Answer from the drawing. Dimensions are ordinates in mm from the lowest x, y and z of the part. A direction names the side the tool comes from. Coordinates: 2 decimals unless noted, no trailing zeros. Write each loop counter-clockwise with the first axis right and the second up, starting at its lowest first coordinate (ties: lowest second). Pieces come first, ordered by that corner, then holes. Notation, with made-up numbers: (40, 11.25) - (73, 11.25) arc R7 ccw to (73, 16.25) - close; hole circle Ø1 at (66, -31). An arc over 180 degrees is marked (long way). Use one line per item in the form item = value. Start each with the question number.
Item 1: Consider probe 1 along X at (y, z) = (28.35, 15); probe 2 along X at (y, z) = (17.5, 4.5); probe 3 along Y at (x, z) = (10.25, 26). Determine where each line is inside the solid, lowest interval first.
Item 2: Determine the mould class of the marked faces 1, 2 and 3 for opening direction X: released by +X, released by -X, zero draft, split by the parting line, or undercut.
Item 3: A cutting plane is placed at A-A (y = 17). Write down the section's boundary in (x, z), then the cut area to 3 significant figures.
Item 4: A cutting plane is placed at C-C (z = 15). Write down the section's boundary in (x, y), then the cut area to 4 significant figures.
Item 5: For the marked faces 4 and 5, determine the directions among +Z, -Z, +X, -X, +Y, -Y from which every point of the face is accessible in a straight line to the end or side of a thin tool.
Item 6: Given pin 1 (8 mm diameter, centred on y = 8, z = 15.5, fed in from +X); pin 2 (8 mm diameter, centred on x = 11, z = 12.5, fed in from -Y), each flat-ended and moving along its own axis, determine where each tip first touches the part or whether it passes through.
Item 7: A cutting plane is placed at D-D (z = 22). Write down the section's boundary in (x, y), then the cut area to 3 significant figures.
Item 8: A cutting plane is placed at B-B (x = 15). Write down the section's boundary in (y, z).
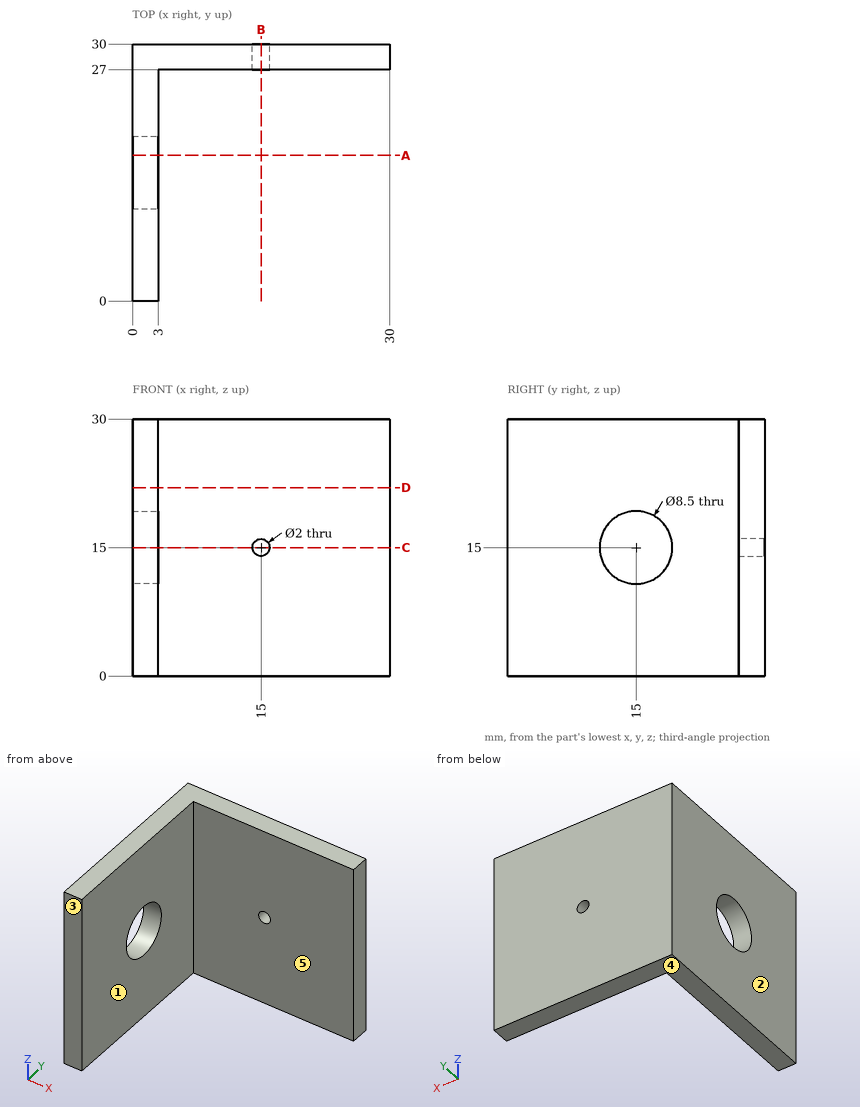
Answer:
q1.probe_1 = 0 to 14, 16 to 30
q1.probe_2 = 0 to 3
q1.probe_3 = 27 to 30
q2.face_1 = released by +X
q2.face_2 = released by -X
q2.face_3 = zero draft
q3.outline = (0, 0) - (3, 0) - (3, 11.25) - (0, 11.25) - close; (0, 18.75) - (3, 18.75) - (3, 30) - (0, 30) - close
q3.area = 67.5 mm²
q4.outline = (0, 0) - (3, 0) - (3, 10.75) - (0, 10.75) - close; (0, 19.25) - (3, 19.25) - (3, 27) - (14, 27) - (14, 30) - (0, 30) - close; (16, 27) - (30, 27) - (30, 30) - (16, 30) - close
q4.area = 139.5 mm²
q5.face_4 = -Z, +X, -X, +Y, -Y
q5.face_5 = +Z, -Z, +X, -Y
q6.pin_1 = 3
q6.pin_2 = 27
q7.outline = (0, 0) - (3, 0) - (3, 27) - (30, 27) - (30, 30) - (0, 30) - close
q7.area = 171 mm²
q8.outline = (27, 0) - (30, 0) - (30, 14) - (27, 14) - close; (27, 16) - (30, 16) - (30, 30) - (27, 30) - close
